from build123d import *

# Parameters (mm, degrees)
SKETCH1_R           = 23.525
SKETCH1_R_2         = 22.525
BOSS_EXTRUDE1_DEPTH = 40
BOSS_EXTRUDE2_DEPTH = 40
SKETCH2_R           = 19.05
CUT_EXTRUDE1_DEPTH  = 59.025
SKETCH4_R           = 15.85
CUT_EXTRUDE2_DEPTH  = 22.144130073


with BuildPart() as part:
    # Sketch1 → Boss-Extrude1 (new body)
    with BuildSketch(Plane.XY):
        Circle(SKETCH1_R)
        Circle(SKETCH1_R_2, mode=Mode.SUBTRACT)
    extrude(amount=-BOSS_EXTRUDE1_DEPTH)

    # Sketch5 → Boss-Extrude2 (add)
    with BuildSketch(Plane(origin=(0, 0, -40), x_dir=(-1, 0, 0), z_dir=(0, 0, -1))):
        with BuildLine():
            ThreePointArc((0, -23.525), (-16.634687027, -16.634687027), (-23.525, 0))
            Line((-23.525, 0), (-23.525, -23.525))
            Line((-23.525, -23.525), (0, -23.525))
        make_face()
        with BuildLine():
            Line((23.525, -23.525), (23.525, 0))
            ThreePointArc((23.525, 0), (16.634687027, -16.634687027), (0, -23.525))
            Line((0, -23.525), (23.525, -23.525))
        make_face()
        Polygon((23.525, -23.525), (23.525, -24.525), (-23.525, -24.525), (-23.525, -23.525), (0, -23.525), align=None)
    extrude(amount=-BOSS_EXTRUDE2_DEPTH)

    # Sketch2 → Cut-Extrude1 (cut, through all)
    with BuildSketch(Plane(origin=(34.5, 0, 0), x_dir=(0, 0, -1), z_dir=(1, 0, 0))):
        Circle(SKETCH2_R)
    extrude(amount=-CUT_EXTRUDE1_DEPTH, mode=Mode.SUBTRACT)

    # Sketch4 → Cut-Extrude2 (cut, through all)
    with BuildSketch(Plane(origin=(0, 0, 0), x_dir=(1, 0, 0), z_dir=(0, -0.898794046, -0.438371147))):
        Circle(SKETCH4_R)
    extrude(amount=-CUT_EXTRUDE2_DEPTH, mode=Mode.SUBTRACT)


solid = part.part
Design review of the part built by this model. Coordinates are the model's own, in mm. A direction names the side the tool comes from. Coordinates: 2 decimals unless noted, no trailing zeros. Order: outer loops, then holes, each group sorted by start corner. A loop starts at its lowest first (then second) coordinate and runs counter-clockwise, first axis right, second up.
Item 1: For line 1 (Y direction, x = 0, z = -21) (3 decimals); line 2 (X direction, y = 0, z = -25) (3 decimals); line 3 (Y direction, x = -2, z = -8) (3 decimals), list the stretches that pass through material, from the lowest coordinate up.
Item 2: The part is to be moulded in two halves that separate along Y. For faces 3 (the flat face through (0, -23, 0)), 4 (the flat face through (0, -24.525, -20)), 5 (the cylindrical face through (-19.45, -15.363, -11.264)), say which applies: pulls with the +Y half, pulls with the -Y half, needs draft (parallel to the pull), parting line crosses it, or undercut.
Item 3: Take a section at C-C, the plane y = -4. Write out the cut boundary in (x, z) (3 decimals), then the cut area to 3 significant figures.
Item 4: For pin 1 Ø8 at (y, z) = (3, -20.5) entering from +X (3 decimals); pin 2 Ø3 at (y, z) = (14, -29.5) entering from -X; pin 3 Ø6 at (y, z) = (15.5, -15.5) entering from +X; pin 4 Ø1.5 at (x, y) = (-16.5, 15.5) entering from +Z, all flat-tipped, find the tip position at first contact; note any pin that passes through.
Item 5: Take a section at B-B, the plane x = 6. Write out the cut boundary in (y, z) (3 decimals), then the cut area to 3 significant figures.
Item 6: For faces 1 (the cylindrical face through (-0.23, 22.7, -6.56)), 2 (the flat face through (0, -24, -40)), list the 3-axis set-ups (+Z, -Z, +X, -X, +Y, -Y) from which the entire face can be reached by the end or side of a thin tool; tool diameter is ignored.
Item 7: Take a section at D-D, the plane z = -31.5. Write out the cut boundary in (x, y) (3 decimals), then the cut area to 3 significant figures.
Item 8: Take a section at A-A, the plane z = -13. Write out the cut boundary in (x, y) (3 decimals).
The answers:
1. line 1: y = -24.525 to -22.525, 22.525 to 23.525
1. line 2: x = -23.525 to -22.525, 22.525 to 23.525
1. line 3: y = -24.525 to -22.436, 22.436 to 23.44
2. face 3: needs draft
2. face 4: pulls with the -Y half
2. face 5: undercut
3. outline: (-23.525, -40) - (-22.167, -40) - (-22.167, -18.625) - (-23.525, -18.625) - close; (22.167, -40) - (23.525, -40) - (23.525, -18.625) - (22.167, -18.625) - close
3. area: 58.1 mm2
4. pin 1: stops at x = 23.525
4. pin 2: stops at x = -19.93
4. pin 3: stops at x = 19.93
4. pin 4: stops at z = -9.94
5. outline: (-24.525, -40) - (-21.711, -40) - (-21.711, 0) - (-24.525, 0) - close; (21.711, -40) - (22.747, -40) - (22.747, -5.228) - (21.711, -5.733) - close
5. area: 148 mm2
6. face 1: +Z
6. face 2: -Z, +X, -X, +Y, -Y
7. outline: (-23.525, -24.525) - (23.525, -24.525) - (23.525, 0) arc R23.525 ccw to (-23.525, 0) - close; hole circle Ø45.05 at (0, 0)
7. area: 429 mm2
8. outline: (-23.525, -24.525) - (23.525, -24.525) - (23.525, -13.925) - (17.705, -13.925) arc R22.525 cw to (-17.705, -13.925) - (-23.525, -13.925) - close; (-18.961, 13.925) - (-17.705, 13.925) arc R22.525 cw to (17.705, 13.925) - (18.961, 13.925) arc R23.525 ccw to start
